Autodesk Inventor part; units mm, degrees
ref_plane "YZ Plane" through (0, 0, 0) normal (1, 0, 0) x (0, 1, 0)
ref_plane "XZ Plane" through (0, 0, 0) normal (0, 1, 0) x (-1, 0, 0)
ref_plane "XY Plane" through (0, 0, 0) normal (0, 0, 1) x (1, 0, 0)
sketch "Sketch1" plane through (0, 0, 0) normal (0, 0, 1) x (1, 0, 0)
  line L0 (-12.7, -25.4) -> (12.7, -25.4)
  line L1 (12.7, -25.4) -> (12.7, 25.4)
  line L2 (12.7, 25.4) -> (-12.7, 25.4)
  line L3 (-12.7, 25.4) -> (-12.7, -25.4)
  line L4 (-12.7, -25.4) -> (12.7, 25.4) construction
  line L5 (12.7, -25.4) -> (-12.7, 25.4) construction
  line L6 (-11.1125, 23.8125) -> (11.1125, 23.8125)
  line L7 (11.1125, 23.8125) -> (11.1125, -23.8125)
  line L8 (11.1125, -23.8125) -> (-11.1125, -23.8125)
  line L9 (-11.1125, -23.8125) -> (-11.1125, 23.8125)
  point P0 (0, 0)
  dimension "width" = 25.4
  dimension "height" = 50.8
  dimension "thickness" = 1.5875
extrude "Extrusion1" add sketch "Sketch1" along normal mid plane 203.2
sketch "Sketch4" plane through (-12.7, 25.4, 101.6) normal (0, 1, 0) x (1, 0, 0)
  line L0 (0, 203.2) -> (25.4, 203.2) construction
  line L1 (25.4, 203.2) -> (25.4, 0) construction
  line L2 (25.4, 0) -> (0, 0) construction
  line L3 (0, 0) -> (0, 203.2) construction
  line L4 (25.4, 0) -> (0, 0)
  line L5 (0, 0) -> (25.4, 25.4)
  line L6 (25.4, 25.4) -> (25.4, 0)
  point P0 (12.7, 101.6)
  dimension "d13" = 45
extrude "Extrusion4" [suppressed]
sketch "Sketch5" plane through (-12.7, 25.4, 101.6) normal (0, 1, 0) x (1, 0, 0)
  line L0 (0, 203.2) -> (25.4, 203.2) construction
  line L1 (25.4, 203.2) -> (25.4, 0) construction
  line L2 (25.4, 0) -> (0, 0) construction
  line L3 (0, 0) -> (0, 203.2) construction
  point P0 (12.7, 101.6)
  point P1 (12.7, 190.5)
  point P2 (12.7, 203.2)
  dimension "d16" = 12.7
hole "Hole1" at (0, 25.4, -88.9) direction (0, -1, 0) diameter 5.1054 end through all
pattern_linear "Rectangular Pattern1" count 8 spacing 25.4 along (0, 0, 1) of "Hole1"
properties part number "CL3-002" material "Aluminum 6061"
Geometry: final body of the model. Coordinates: model frame, mm. A direction names the side the tool comes from. Give positions to 0.01 mm unless a question says otherwise; leave off trailing zeros. Order: outer loops, then holes, each group sorted by start corner. A loop starts at its lowest first (then second) coordinate and runs counter-clockwise, first axis right, second up. Notation, with made-up numbers: M -7.5,20 L 29.5,20 A10 ccw 29.5,27 Z; hole C -16,7 d3. An arc over 180 degrees is marked long. Answer as CSV lines item,"result". Start each with the question number.
1) Cut plane B-B (x = -6.25). Output: boundary loops of the cut face in (y, z).
2) Cut plane A-A (z = 63.5). Output: boundary loops of the cut face in (x, y), then the cut area to 3 significant figures.
3) Set-up query: faces 3 (the flat face through (11.112, 0, -1)), 4 (the cylindrical face through (-0.11, 24.6, -66.05)). Return all of +Z, -Z, +X, -X, +Y, -Y with unobstructed straight access to the full face (end or side cutting, diameter ignored); none if empty.
4) Mould query, pull axis X, two halves, no side actions, for faces 1 (the flat face through (-11.3, 2, -101.6)), 2 (the flat face through (0, 23.812, -1)). Classes: +X half, -X half, draft (parallel to the pull), parting line (faces both ways), or undercut.
5) Line query: line 1 (X direction, y = 16.5, z = 36.5); line 2 (Y direction, x = -7, z = 51.5); line 3 (X direction, y = 24.7, z = 38.1). Output: solid intervals per line, ascending. Write a range as from..to.
6) Cut plane D-D (z = -4.5). Output: boundary loops of the cut face in (x, y), then the cut area to 3 significant figures.
7) Cut plane C-C (y = 5). Output: boundary loops of the cut face in (x, z).
Findings below:
1,outline,"M -25.4,-101.6 L -23.81,-101.6 L -23.81,101.6 L -25.4,101.6 Z; M 23.81,-101.6 L 25.4,-101.6 L 25.4,101.6 L 23.81,101.6 Z"
2,outline,"M -12.7,-25.4 L -2.55,-25.4 L -2.55,-23.81 L -11.11,-23.81 L -11.11,23.81 L -2.55,23.81 L -2.55,25.4 L -12.7,25.4 Z; M 2.55,-25.4 L 12.7,-25.4 L 12.7,25.4 L 2.55,25.4 L 2.55,23.81 L 11.11,23.81 L 11.11,-23.81 L 2.55,-23.81 Z"
2,area,"216 mm²"
3,face 3,"+Z, -Z"
3,face 4,"+Y, -Y"
4,face 1,"draft"
4,face 2,"undercut"
5,line 1,"x = -12.7..-11.11, 11.11..12.7"
5,line 2,"y = -25.4..-23.81, 23.81..25.4"
5,line 3,"x = -12.7..-2.55, 2.55..12.7"
6,outline,"M -12.7,-25.4 L 12.7,-25.4 L 12.7,25.4 L -12.7,25.4 Z; hole M -11.11,-23.81 L 11.11,-23.81 L 11.11,23.81 L -11.11,23.81 Z"
6,area,"232 mm²"
7,outline,"M -12.7,-101.6 L -11.11,-101.6 L -11.11,101.6 L -12.7,101.6 Z; M 11.11,-101.6 L 12.7,-101.6 L 12.7,101.6 L 11.11,101.6 Z"
